```python
from build123d import *

# Parameters (mm, degrees)
F0_R           = 2.8
F0_R_2         = 1.5
F1_DEPTH       = 6
F2_DEPTH       = 5
F3_D           = 5.5
F3_DEPTH       = 30
F3_CBORE_D     = 9.5
F3_CBORE_DEPTH = 1.5
F3_TIP         = 1.6523667023
F5_D           = 2.8
F5_CBORE_D     = 4
F5_CBORE_DEPTH = 4
F6_W           = 35
F6_H           = 17
F6_H_2         = 6
F7_DEPTH       = 8
F7_DEPTH_BACK  = 0.4
F10_DEPTH      = 3.7
F10_DEPTH_BACK = 2.5
F11_D          = 7
F11_DEPTH      = 4.201
F13_D          = 2.8


with BuildPart() as f1:
    # F0 (on Top) → F1 (new body)
    with BuildSketch(Plane.XY):
        with BuildLine():
            Line((-6, 17.5), (-17.5, 17.5))
            Line((-17.5, 17.5), (-17.5, -17.5))
            Line((-17.5, -17.5), (17.5, -17.5))
            Line((17.5, -17.5), (17.5, 17.5))
            Line((17.5, 17.5), (6, 17.5))
            Line((6, 17.5), (3.3166247904, 17.5))
            ThreePointArc((3.3166247904, 17.5), (0, 16.5), (-3.3166247904, 17.5))
            Line((-3.3166247904, 17.5), (-6, 17.5))
        make_face()
        with Locations((-14, -14)):
            Circle(F0_R, mode=Mode.SUBTRACT)
        with Locations((-14, -3.75)):
            Circle(F0_R_2, mode=Mode.SUBTRACT)
        with Locations((-14, 3.75)):
            Circle(F0_R_2, mode=Mode.SUBTRACT)
        with Locations((14, -14)):
            Circle(F0_R, mode=Mode.SUBTRACT)
        with Locations((14, -3.75)):
            Circle(F0_R_2, mode=Mode.SUBTRACT)
        with Locations((14, 3.75)):
            Circle(F0_R_2, mode=Mode.SUBTRACT)
        with Locations((-14, 14)):
            Circle(F0_R, mode=Mode.SUBTRACT)
        with Locations((14, 14)):
            Circle(F0_R, mode=Mode.SUBTRACT)
        with BuildLine():
            ThreePointArc((-6, 22.5), (-5.2867640737, 19.6627256691), (-3.3166247904, 17.5))
            Line((-3.3166247904, 17.5), (3.3166247904, 17.5))
            ThreePointArc((3.3166247904, 17.5), (5.2867640737, 19.6627256691), (6, 22.5))
            Line((6, 22.5), (-6, 22.5))
        make_face()
        with BuildLine():
            ThreePointArc((6, 22.5), (0, 28.5), (-6, 22.5))
            Line((-6, 22.5), (6, 22.5))
        make_face()
        with BuildLine():
            ThreePointArc((6, 22.5), (5.2867640737, 19.6627256691), (3.3166247904, 17.5))
            Line((3.3166247904, 17.5), (6, 17.5))
            Line((6, 17.5), (6, 22.5))
        make_face()
        with BuildLine():
            Line((3.3166247904, 17.5), (-3.3166247904, 17.5))
            ThreePointArc((-3.3166247904, 17.5), (0, 16.5), (3.3166247904, 17.5))
        make_face()
        with BuildLine():
            Line((-6, 22.5), (-6, 17.5))
            Line((-6, 17.5), (-3.3166247904, 17.5))
            ThreePointArc((-3.3166247904, 17.5), (-5.2867640737, 19.6627256691), (-6, 22.5))
        make_face()
        with Locations((-14, -14)):
            Circle(F0_R)
        with Locations((14, -14)):
            Circle(F0_R)
        with Locations((14, 14)):
            Circle(F0_R)
        with Locations((-14, 14)):
            Circle(F0_R)
        with Locations((-14, 3.75)):
            Circle(F0_R_2)
        with Locations((-14, -3.75)):
            Circle(F0_R_2)
        with Locations((14, -3.75)):
            Circle(F0_R_2)
        with Locations((14, 3.75)):
            Circle(F0_R_2)
    extrude(amount=F1_DEPTH)

    # F0 (on Top) → F2 (join)
    with BuildSketch(Plane.XY):
        with Locations((-14, -14)):
            Circle(F0_R)
        with Locations((-14, 14)):
            Circle(F0_R)
        with Locations((14, 14)):
            Circle(F0_R)
        with Locations((14, -14)):
            Circle(F0_R)
        with Locations((-14, 3.75)):
            Circle(F0_R_2)
        with Locations((-14, -3.75)):
            Circle(F0_R_2)
        with Locations((14, -3.75)):
            Circle(F0_R_2)
        with Locations((14, 3.75)):
            Circle(F0_R_2)
    extrude(amount=-F2_DEPTH)

    # F3
    with Locations(Plane(origin=(0, 0, 0), x_dir=(1, 0, 0), z_dir=(0, 0, -1))):
        with Locations((0, -22.5)):
            CounterBoreHole(F3_D / 2, F3_CBORE_D / 2, F3_CBORE_DEPTH, depth=F3_DEPTH)
            with Locations((0, 0, -(F3_DEPTH + F3_TIP / 2))):  # 118° drill point
                Cone(0, F3_D / 2, F3_TIP, mode=Mode.SUBTRACT)

    # F5 (through all)
    with Locations(Plane.XY.offset(6)):
        with Locations((-14, 14), (14, 14), (14, -14), (-14, -14)):
            CounterBoreHole(F5_D / 2, F5_CBORE_D / 2, F5_CBORE_DEPTH)

    # F6 (on face) → F7 (join, two sides)
    with BuildSketch(Plane.XZ.offset(17.5)) as f7_sk:
        with Locations((0, -8.5)):
            Rectangle(F6_W, F6_H)
        with Locations((0, 3)):
            Rectangle(F6_W, F6_H_2)
    extrude(amount=F7_DEPTH)
    extrude(f7_sk.sketch, amount=-F7_DEPTH_BACK)

    # F9 (on mid) → F10 (cut, two sides)
    with BuildSketch(Plane(origin=(0, -21.3, 0), x_dir=(-1, 0, 0), z_dir=(0, 1, 0))) as f10_sk:
        Polygon((5.562, -13.7887778028), (-5.562, -13.7887778028), (0, -17), align=None)
        Polygon((-5.562, -7.3663334083), (-5.562, -13.7887778028), (5.562, -13.7887778028), (5.562, -7.3663334083), (0, -4.1551112111), align=None)
        Polygon((0, -17), (-5.562, -13.7887778028), (-5.562, -17), align=None)
        Polygon((5.562, -13.7887778028), (0, -17), (5.562, -17), align=None)
    extrude(amount=F10_DEPTH, mode=Mode.SUBTRACT)
    extrude(f10_sk.sketch, amount=-F10_DEPTH_BACK, mode=Mode.SUBTRACT)

    # F11 (through all, one way)
    with BuildSketch(Plane(origin=(0, -21.3, 0), x_dir=(-1, 0, 0), z_dir=(0, 1, 0))):
        with Locations((0, -10.5775556055)):
            Circle(F11_D / 2)
    extrude(amount=-F11_DEPTH, mode=Mode.SUBTRACT)

    # F13 (through all)
    with Locations(Plane.XY.offset(6)):
        with Locations((0, -21.3)):
            Hole(F13_D / 2)


solid = f1.part
```
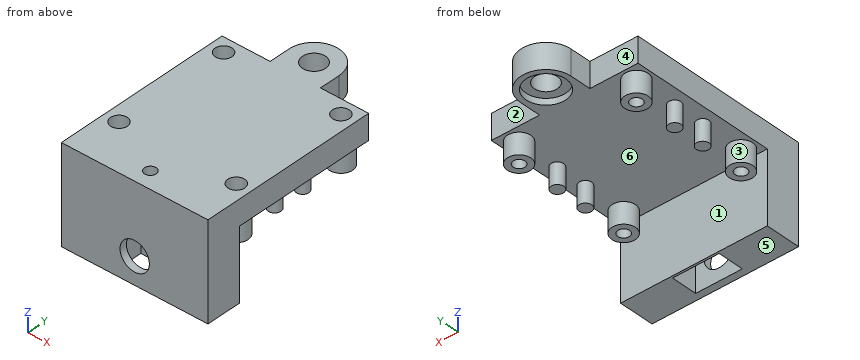
Can you work these out from the model? Positions are in its coordinate system, mm. Face numbers are marked on the shaded views. A direction names the side the tool comes from. Round coordinates to 2 decimals unless told otherwise and drop trailing zeros. Loops run counter-clockwise (first coordinate to the right, second up) from the corner with the lowest first, then second, coordinate; pieces in that order, holes last. Notation, with made-up numbers: M 51.25,65 L 66.25,65 A14 cw 66.25,79 Z; hole C -36,65 d1. An arc over 180 degrees is marked long. Answer as a JSON object with one key per item and string values. Group by question number.
Q1. Imagine slicing it at D-D, the plane y = -3.75. Please give me the cut outline in (x, z).
Q2. Will these pins go through, and if not, where does the flat tip stop? pin 1 (4.5 mm diameter, centred on x = 14, y = -14, fed in from +Z); pin 2 (2.5 mm diameter, centred on x = 14.5, y = -3.5, fed in from -Z); pin 3 (1 mm diameter, centred on x = 7.5, z = -13.5, fed in from +Y); pin 4 (1.5 mm diameter, centred on x = -7.5, y = 17.5, fed in from -Z).
Q3. Imagine slicing it at C-C, the plane z = 3.25. Please give me the cut outline in (x, y), then the cut area to 3 significant figures.
Q4. We'd pull the mould along Y, two halves only. Please class the marked faces 4, 5 and 6: +Y half, -Y half, draft (parallel to the pull), parting line (faces both ways), or undercut.
Q5. On a 3-axis mill with a long thin cutter (end or side, diameter ignored), from which of +Z, -Z, +X, -X, +Y, -Y can I reach the whole of each face in a straight line? I mean the marked faces 1, 2 and 3. Say none if no direction works.
Q6. Imagine slicing it at A-A, the plane x = 2. Please give me the cut outline in (y, z).
Q7. Please list where these lines run through material, in increasing order: L1, parallel to Y at x = -14, z = 3.2; L2, parallel to Y at x = -9, z = 2.5; L3, parallel to Z at x = 4.5, y = -3.
Q8. Imagine slicing it at B-B, the plane y = -14. Please give me the cut outline in (x, z), then the cut area to 3 significant figures.
Findings:
{
 "1": {"outline": "M -17.5,0 L -15.5,0 L -15.5,-5 L -12.5,-5 L -12.5,0 L 12.5,0 L 12.5,-5 L 15.5,-5 L 15.5,0 L 17.5,0 L 17.5,6 L -17.5,6 Z"},
 "2": {"pin 1": "stops at z = 6", "pin 2": "stops at z = -5", "pin 3": "stops at y = -17.1", "pin 4": "stops at z = 0"},
 "3": {"outline": "M -17.5,-25.5 L 17.5,-25.5 L 17.5,17.5 L 6,17.5 L 6,22.5 A6 ccw -6,22.5 L -6,17.5 L -17.5,17.5 Z; hole C -14,-14 d4; hole C -14,14 d4; hole C 0,22.5 d5.5; hole C 0,-21.3 d2.8; hole C 14,-14 d4; hole C 14,14 d4", "area": "1,540 mm2"},
 "4": {"face 4": "+Y half", "face 5": "draft", "face 6": "undercut"},
 "5": {"face 1": "-Z, +X, -X", "face 2": "+Z, -Z, +X, +Y", "face 3": "-Z"},
 "6": {"outline": "M -25.5,-17 L -23.8,-17 L -23.8,-13.45 L -25.5,-13.45 Z; M -25.5,-7.71 L -23.8,-7.71 L -23.8,-5.31 L -17.6,-5.31 L -17.6,-17 L -17.1,-17 L -17.1,0 L 18.19,0 L 18.19,1.5 L 20.61,1.5 L 20.61,6 L -25.5,6 Z; M 24.39,1.5 L 26.81,1.5 L 26.81,0 L 28.16,0 L 28.16,6 L 24.39,6 Z"},
 "7": {"L1": "y = -25.5 to -16, -12 to 12, 16 to 17.5", "L2": "y = -25.5 to 17.5", "L3": "z = 0 to 6"},
 "8": {"outline": "M -17.5,0 L -16.8,0 L -16.8,-5 L -15.4,-5 L -15.4,2 L -16,2 L -16,6 L -17.5,6 Z; M -12.6,-5 L -11.2,-5 L -11.2,0 L 11.2,0 L 11.2,-5 L 12.6,-5 L 12.6,2 L 12,2 L 12,6 L -12,6 L -12,2 L -12.6,2 Z; M 15.4,-5 L 16.8,-5 L 16.8,0 L 17.5,0 L 17.5,6 L 16,6 L 16,2 L 15.4,2 Z", "area": "195 mm2"}
}
